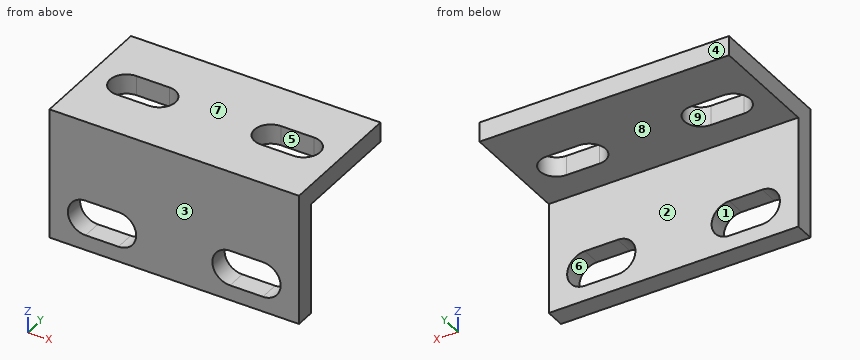
from build123d import *

# Parameters (mm, degrees)
BOSS_EXTRUDE1_DEPTH = 38
CUT_EXTRUDE1_DEPTH  = 4
CUT_EXTRUDE2_DEPTH  = 4


with BuildPart() as part:
    # Sketch1 → Boss-Extrude1 (new body)
    with BuildSketch(Plane(origin=(0, 0, 0), x_dir=(0, 0, -1), z_dir=(1, 0, 0))):
        Polygon((0, 0), (-17, 0), (-17, 17), (-20, 17), (-20, -3), (0, -3), align=None)
    extrude(amount=BOSS_EXTRUDE1_DEPTH)

    # Sketch2 → Cut-Extrude1 (cut)
    with BuildSketch(Plane(origin=(0, 0, 0), x_dir=(1, 0, 0), z_dir=(0, 1, 0))):
        with BuildLine():
            Line((5.5, -2.3), (10.5, -2.3))
            ThreePointArc((10.5, -2.3), (13.2, -5), (10.5, -7.7))
            Line((10.5, -7.7), (5.5, -7.7))
            ThreePointArc((5.5, -7.7), (2.8, -5), (5.5, -2.3))
        make_face()
        with BuildLine():
            Line((32.5, -2.3), (27.5, -2.3))
            ThreePointArc((27.5, -2.3), (24.8, -5), (27.5, -7.7))
            Line((27.5, -7.7), (32.5, -7.7))
            ThreePointArc((32.5, -7.7), (35.2, -5), (32.5, -2.3))
        make_face()
    extrude(amount=-CUT_EXTRUDE1_DEPTH, mode=Mode.SUBTRACT)

    # Sketch3 → Cut-Extrude2 (cut)
    with BuildSketch(Plane(origin=(0, 0, 17), x_dir=(-1, 0, 0), z_dir=(0, 0, -1))):
        with BuildLine():
            Line((-32.5, 9.5), (-27.5, 9.5))
            ThreePointArc((-27.5, 9.5), (-25, 7), (-27.5, 4.5))
            Line((-27.5, 4.5), (-32.5, 4.5))
            ThreePointArc((-32.5, 4.5), (-35, 7), (-32.5, 9.5))
        make_face()
        with BuildLine():
            Line((-5.5, 9.5), (-10.5, 9.5))
            ThreePointArc((-10.5, 9.5), (-13, 7), (-10.5, 4.5))
            Line((-10.5, 4.5), (-5.5, 4.5))
            ThreePointArc((-5.5, 4.5), (-3, 7), (-5.5, 9.5))
        make_face()
    extrude(amount=-CUT_EXTRUDE2_DEPTH, mode=Mode.SUBTRACT)


solid = part.part
Geometry: final body of the model. Coordinates: model frame, mm. Face numbers are marked on the shaded views. A direction names the side the tool comes from. Give positions to 0.01 mm unless a question says otherwise; leave off trailing zeros. Order: outer loops, then holes, each group sorted by start corner. A loop starts at its lowest first (then second) coordinate and runs counter-clockwise, first axis right, second up. Notation, with made-up numbers: (-5, -38) -> (9, -38) arc R20 ccw to (9, -7) -> close; hole circle Ø4 at (45.25, 75.5). An arc over 180 degrees is marked (long way). Put each result on its own line as item: value.
Q1. Reachability of the marked faces 1, 2, 3, 4 and 5 from +Z, -Z, +X, -X, +Y, -Y: full face, straight path, thin tool, end or side. Return the list, or none.
Here are the results:
face 1: +Y, -Y
face 2: -Z, +X, -X, +Y
face 3: +Z, -Z, +X, -X, -Y
face 4: +Z, -Z, +X, -X, +Y
face 5: +Z, -Z
Q2. Section D-D, the plane x = 5. Return loops of the section in (y, z).
Here are the results:
outline: (-3, 0) -> (0, 0) -> (0, 2.35) -> (-3, 2.35) -> close; (-3, 7.65) -> (0, 7.65) -> (0, 17) -> (4.55, 17) -> (4.55, 20) -> (-3, 20) -> close; (9.45, 17) -> (17, 17) -> (17, 20) -> (9.45, 20) -> close
Q3. Section B-B, the plane x = 30. Return loops of the section in (y, z).
Here are the results:
outline: (-3, 0) -> (0, 0) -> (0, 2.3) -> (-3, 2.3) -> close; (-3, 7.7) -> (0, 7.7) -> (0, 17) -> (4.5, 17) -> (4.5, 20) -> (-3, 20) -> close; (9.5, 17) -> (17, 17) -> (17, 20) -> (9.5, 20) -> close
Q4. Pin query (flat end, axial travel): pin 1 (3 mm diameter, centred on x = 13.5, y = 8.5, fed in from -Z); pin 2 (8.5 mm diameter, centred on x = 26, z = 6.5, fed in from +Y). Return the tip coordinate at first contact, or that it passes through.
Here are the results:
pin 1: stops at z = 17
pin 2: stops at y = 0
Q5. Material intervals for L1, parallel to X at y = -1, z = 5.5; L2, parallel to Z at x = 16.5, y = 13.75; L3, parallel to Y at x = 3, z = 12.75, sorted ascending.
Here are the results:
L1: x = 0 to 2.85, 13.15 to 24.85, 35.15 to 38
L2: z = 17 to 20
L3: y = -3 to 0
Q6. Section A-A, the plane z = 5. Return loops of the section in (x, y), then the cut area to 3 significant figures.
Here are the results:
outline: (0, -3) -> (2.8, -3) -> (2.8, 0) -> (0, 0) -> close; (13.2, -3) -> (24.8, -3) -> (24.8, 0) -> (13.2, 0) -> close; (35.2, -3) -> (38, -3) -> (38, 0) -> (35.2, 0) -> close
area: 51.6 mm^2
Q7. Section C-C, the plane y = 7. Return loops of the section in (x, z).
Here are the results:
outline: (0, 17) -> (3, 17) -> (3, 20) -> (0, 20) -> close; (13, 17) -> (25, 17) -> (25, 20) -> (13, 20) -> close; (35, 17) -> (38, 17) -> (38, 20) -> (35, 20) -> close
Q8. Draft query along Z for the marked faces 6, 7, 8 and 9. Return one class per face: released by +Z, released by -Z, zero draft, split by the parting line, or undercut.
Here are the results:
face 6: undercut
face 7: released by +Z
face 8: released by -Z
face 9: zero draft
